from build123d import *

# Parameters (mm, degrees)
F3_DEPTH = 10.001


with BuildPart() as f1:
    # F0 (on Front) → F1 (revolve)
    with BuildSketch(Plane.XZ):
        Polygon((20, 25), (15, 25), (15, 0), (45, 0), (45, 10), (20, 10), align=None)
    revolve(axis=Axis((0, 0, 17.8506122556), (0, 0, -1)))

    # F2 (on face) → F3 (cut, through all)
    with BuildSketch(Plane.XY.offset(10)):
        with BuildLine():
            ThreePointArc((29.0030388795, 14.6653924514), (26.1540541981, 8.4979673453), (32.0840527441, 5.1830068027))
            ThreePointArc((32.0840527441, 5.1830068027), (30.9093367796, 10.0430523172), (29.0030388795, 14.6653924514))
        make_face()
        with BuildLine():
            ThreePointArc((29.0030388795, 14.6653924514), (30.9093367796, 10.0430523172), (32.0840527441, 5.1830068027))
            ThreePointArc((32.0840527441, 5.1830068027), (34.8383048262, 6.9506082855), (35.9093367796, 10.0430523172))
            ThreePointArc((35.9093367796, 10.0430523172), (33.6903896827, 14.1982592615), (29.0030388795, 14.6653924514))
        make_face()
        with BuildLine():
            ThreePointArc((24.1030206995, -26.2930523172), (23.7953091225, -24.5660811664), (22.9100489572, -23.0516736221))
            ThreePointArc((22.9100489572, -23.0516736221), (19.1030206995, -26.2930523172), (14.84384994, -28.9121102474))
            ThreePointArc((14.84384994, -28.9121102474), (20.4639296242, -31.1042815675), (24.1030206995, -26.2930523172))
        make_face()
        with BuildLine():
            ThreePointArc((14.84384994, -28.9121102474), (19.1030206995, -26.2930523172), (22.9100489572, -23.0516736221))
            ThreePointArc((22.9100489572, -23.0516736221), (16.164094438, -22.2479673453), (14.84384994, -28.9121102474))
        make_face()
        with BuildLine():
            ThreePointArc((-4.9851851526, 32.1153846154), (0, 27.5), (4.9851851526, 32.1153846154))
            ThreePointArc((4.9851851526, 32.1153846154), (0, 32.5), (-4.9851851526, 32.1153846154))
        make_face()
        with BuildLine():
            ThreePointArc((-4.9851851526, 32.1153846154), (0, 32.5), (4.9851851526, 32.1153846154))
            ThreePointArc((4.9851851526, 32.1153846154), (4.9962949154, 32.3075496988), (5, 32.5))
            ThreePointArc((5, 32.5), (-0.1924503012, 37.4962949154), (-4.9851851526, 32.1153846154))
        make_face()
        with BuildLine():
            ThreePointArc((-22.9100489572, -23.0516736221), (-22.041946961, -30.3381372891), (-14.84384994, -28.9121102474))
            ThreePointArc((-14.84384994, -28.9121102474), (-19.1030206995, -26.2930523172), (-22.9100489572, -23.0516736221))
        make_face()
        with BuildLine():
            ThreePointArc((-22.9100489572, -23.0516736221), (-19.1030206995, -26.2930523172), (-14.84384994, -28.9121102474))
            ThreePointArc((-14.84384994, -28.9121102474), (-14.2917914492, -27.6539612419), (-14.1030206995, -26.2930523172))
            ThreePointArc((-14.1030206995, -26.2930523172), (-17.3760495487, -21.6007638942), (-22.9100489572, -23.0516736221))
        make_face()
        with BuildLine():
            ThreePointArc((-25.9093367796, 10.0430523172), (-26.7541298353, 12.8241052203), (-29.0030388795, 14.6653924514))
            ThreePointArc((-29.0030388795, 14.6653924514), (-30.9093367796, 10.0430523172), (-32.0840527441, 5.1830068027))
            ThreePointArc((-32.0840527441, 5.1830068027), (-27.8168927479, 6.1140842706), (-25.9093367796, 10.0430523172))
        make_face()
        with BuildLine():
            ThreePointArc((-32.0840527441, 5.1830068027), (-30.9093367796, 10.0430523172), (-29.0030388795, 14.6653924514))
            ThreePointArc((-29.0030388795, 14.6653924514), (-35.6646193611, 11.5881372891), (-32.0840527441, 5.1830068027))
        make_face()
    extrude(amount=-F3_DEPTH, mode=Mode.SUBTRACT)


solid = f1.part
Check sheet for the modelled part. Datum: model origin and axes. Units: mm. A direction names the side the tool comes from. Give positions to 0.01 mm unless a question says otherwise; leave off trailing zeros. Loops run counter-clockwise (first coordinate to the right, second up) from the corner with the lowest first, then second, coordinate; pieces in that order, holes last. Notation, with made-up numbers: M -5,74 L 45,74 A7 cw 45,79 Z; hole C 85.25,-17 d6. An arc over 180 degrees is marked long. Answer as a JSON object with one key per item and string values. Group by question number.
Q1. Cross-section at A-A on x = 0. Record the cut outline in (y, z), then the cut area to 3 significant figures.
Q2. Release check for a two-part mould opening along X. For faces 3 (the cylindrical face through (20.765, 39.923, 5.07)), 4 (the cylindrical face through (-14.985, -0.66, 12.325)), 5 (the flat face through (9, 19, 10)) record: released by +X, released by -X, zero draft, split by the parting line, or undercut.
Q3. Cross-section at D-D on z = 18.25. Record the cut outline in (x, y).
Q4. Cross-section at B-B on y = 0. Record the cut outline in (x, z), then the cut area to 3 significant figures.
Q5. Go/stop test with flat-tipped pins: P1, Ø4, axis at x = 7.5, z = 20.5, coming from the -Y side; P2, Ø4, axis at y = 16.5, z = 9.5, coming from the +X side; P3, Ø1.5, axis at y = -16, z = 7, coming from the +X side. Record where each tip stops, or that it passes through.
Q6. Material ranges on line 1 along X through (y, z) = (0, 12.25); line 2 along X through (y, z) = (0, 8.5), recorded low to high. Write a range as [from, to].
Q7. Cross-section at C-C on x = -17.5. Record the cut outline in (y, z), then the cut area to 3 significant figures.
Q8. Access from +Z, -Z, +X, -X, +Y, -Y to the whole of each face (thin tool, end or side, straight path). Record for faces 1 (the cylindrical face through (-4.336, 19.524, 17.605)), 2 (the flat face through (3, -15, 25)).
Evaluation:
{
 "1": {"outline": "M -45,0 L -15,0 L -15,25 L -20,25 L -20,10 L -45,10 Z; M 15,0 L 27.5,0 L 27.5,10 L 20,10 L 20,25 L 15,25 Z; M 37.5,0 L 45,0 L 45,10 L 37.5,10 Z", "area": "650 mm2"},
 "2": {"face 3": "split by the parting line", "face 4": "undercut", "face 5": "zero draft"},
 "3": {"outline": "C 0,0 d40; hole C 0,0 d30"},
 "4": {"outline": "M -45,0 L -15,0 L -15,25 L -20,25 L -20,10 L -45,10 Z; M 15,0 L 45,0 L 45,10 L 20,10 L 20,25 L 15,25 Z", "area": "750 mm2"},
 "5": {"P1": "stops at y = -19.23", "P2": "stops at x = 42.6", "P3": "stops at x = 42.34"},
 "6": {"line 1": "x = [-20, -15], [15, 20]", "line 2": "x = [-45, -15], [15, 45]"},
 "7": {"outline": "M -41.46,0 L -31.03,0 L -31.03,10 L -41.46,10 Z; M -21.56,0 L 41.46,0 L 41.46,10 L 9.68,10 L 9.68,25 L -9.68,25 L -9.68,10 L -21.56,10 Z", "area": "1,020 mm2"},
 "8": {"face 1": "+Z", "face 2": "+Z, +X, -X, +Y, -Y"}
}
